Can you work these out from the model? Positions are in its coordinate system, mm. Give positions to 0.01 mm unless a question says otherwise; leave off trailing zeros. Order: outer loops, then holes, each group sorted by start corner. A loop starts at its lowest first (then second) coordinate and runs counter-clockwise, first axis right, second up. Notation, with made-up numbers: (-35, 68) - (13, 68) arc R19 cw to (13, 90) - close; hole circle Ø9 at (67.5, 23). An arc over 180 degrees is marked (long way). Return JSON: item names as keys, results as strings.
```python
from build123d import *

# Parameters (mm, degrees)
CROQUIS1_R              = 31.75
SALIENTE_EXTRUIR1_DEPTH = 1000
SALIENTE_EXTRUIR2_DEPTH = 1000


with BuildPart() as part:
    # Croquis1 → Saliente-Extruir1 (new body)
    with BuildSketch(Plane.XY):
        Circle(CROQUIS1_R)
    extrude(amount=SALIENTE_EXTRUIR1_DEPTH)

    # Croquis2 → Saliente-Extruir2 (add)
    with BuildSketch(Plane.XY.offset(1000)):
        Polygon((31.75, 0), (31.75, -1), (30.75, -1), (30.75, 1), (31.75, 1), align=None)
        Polygon((-31.75, 1), (-31.75, 0), (-31.75, -1), (-30.75, -1), (-30.75, 1), align=None)
        Polygon((0, 31.75), (1, 31.75), (1, 30.75), (-1, 30.75), (-1, 31.75), align=None)
        Polygon((-1, -31.75), (0, -31.75), (1, -31.75), (1, -30.75), (-1, -30.75), align=None)
    extrude(amount=-SALIENTE_EXTRUIR2_DEPTH)


solid = part.part
```
1. For pin 1 Ø5 at (y, z) = (20, 542) entering from -X; pin 2 Ø2 at (y, z) = (1.5, 653) entering from +X; pin 3 Ø2 at (y, z) = (23, 591) entering from -X; pin 4 Ø2 at (y, z) = (-25, 431) entering from +X, each with a flat end and sliding along its axis, tell me the tip position at first contact or that it passes through.
Checks:
{"pin 1": "x = -26.49", "pin 2": "x = 31.75", "pin 3": "x = -22.89", "pin 4": "x = 20.79"}
2. Suppose I cut it at B-B (x = -10.5). List the corners of the cut face in (y, z) for me.
Checks:
{"outline": "(-29.96, 0) - (29.96, 0) - (29.96, 1000) - (-29.96, 1000) - close"}
3. If I drill on L1, parallel to Y at x = -3.5, z = 488.5; L2, parallel to Y at x = -27, z = 290.5, over which ranges is the centre line in solid material (lowest first)? Write a range as [from, to].
Checks:
{"L1": "[-31.56, 31.56]", "L2": "[-16.71, 16.71]"}
4. Suppose I cut it at C-C (y = -15.5). List the corners of the cut face in (x, z) for me, plus the area to 3 significant figures.
Checks:
{"outline": "(-27.71, 0) - (27.71, 0) - (27.71, 1000) - (-27.71, 1000) - close", "area": "55,400 mm^2"}
